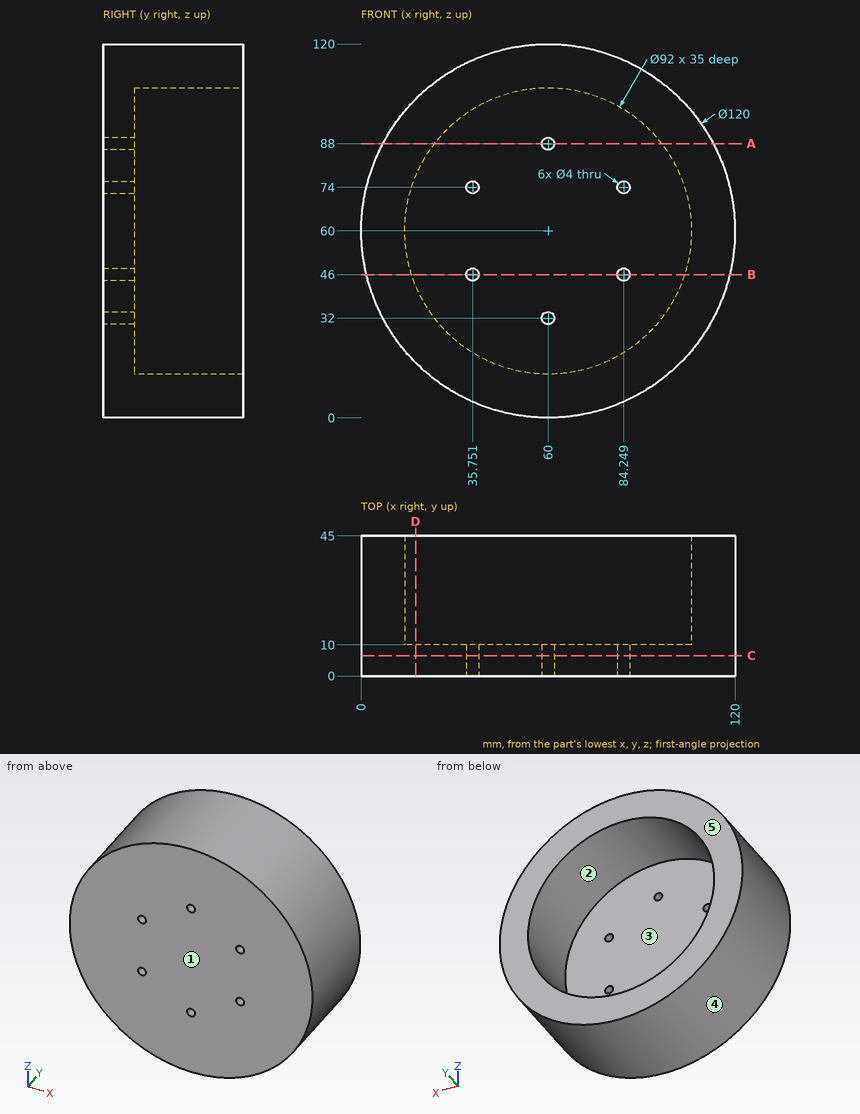
Print and shaded views of the part. All mm, measured from the part's lowest x, y and z. A direction names the side the tool comes from. Round coordinates to 2 decimals unless told otherwise and drop trailing zeros. Write each loop counter-clockwise with the first axis right and the second up, starting at its lowest first coordinate (ties: lowest second). Pieces come first, ordered by that corner, then holes. Notation, with made-up numbers: (87, 37.25) - (98, 37.25) arc R15 ccw to (98, 62.25) - close; hole circle Ø6 at (8.25, 46). An arc over 180 degrees is marked (long way). One line per item, written item: value.
(1) Cut at C-C, the plane y = 6.5. Give the cut face in (x, z), plus the area to 3 significant figures.
Values follow:
outline: circle Ø120 at (60, 60); hole circle Ø4 at (35.75, 46); hole circle Ø4 at (35.75, 74); hole circle Ø4 at (60, 32); hole circle Ø4 at (60, 88); hole circle Ø4 at (84.25, 46); hole circle Ø4 at (84.25, 74)
area: 11,200 mm²
(2) Drop flat-ended pins along their axis: P1, Ø3, axis at x = 60, z = 88, coming from the -Y side; P2, Ø4, axis at x = 36.5, z = 37, coming from the +Y side; P3, Ø1, axis at x = 80.5, y = 30, coming from the +Z side; P4, Ø1.5, axis at y = 32, z = 57.5, coming from the -X side. Give the stop position or say it passes through.
Values follow:
P1: passes through
P2: stops at y = 10
P3: stops at z = 116.57
P4: stops at x = 0.03
(3) Cut at D-D, the plane x = 17.5. Give the cut face in (y, z).
Values follow:
outline: (0, 17.65) - (45, 17.65) - (45, 42.4) - (10, 42.4) - (10, 77.6) - (45, 77.6) - (45, 102.35) - (0, 102.35) - close
(4) Cut at A-A, the plane z = 88. Give the cut face in (x, y), plus the area to 3 significant figures.
Values follow:
outline: (6.93, 0) - (58, 0) - (58, 10) - (23.5, 10) - (23.5, 45) - (6.93, 45) - close; (62, 0) - (113.07, 0) - (113.07, 45) - (96.5, 45) - (96.5, 10) - (62, 10) - close
area: 2,180 mm²
(5) Wall check: probe 1 along X at (y, z) = (5.5, 74); probe 2 along X at (y, z) = (28, 60); probe 3 along Y at (x, z) = (74.5, 37.5). Give the ranges that are in metal, low to high.
Values follow:
probe 1: x = 1.66 to 33.75, 37.75 to 82.25, 86.25 to 118.34
probe 2: x = 0 to 14, 106 to 120
probe 3: y = 0 to 10
(6) Two-plate mould, pull along Z, no slides. Class the marked faces 3, 4 and 5: pulls with the +Z half, pulls with the -Z half, needs draft (parallel to the pull), parting line crosses it, or undercut.
Values follow:
face 3: undercut
face 4: parting line crosses it
face 5: needs draft
(7) Cut at B-B, the plane z = 46. Give the cut face in (x, y).
Values follow:
outline: (1.66, 0) - (33.75, 0) - (33.75, 10) - (16.18, 10) - (16.18, 45) - (1.66, 45) - close; (37.75, 0) - (82.25, 0) - (82.25, 10) - (37.75, 10) - close; (86.25, 0) - (118.34, 0) - (118.34, 45) - (103.82, 45) - (103.82, 10) - (86.25, 10) - close
(8) 3-axis set-ups, long thin cutter, end or side, ignore diameter. For the marked faces 1 and 2: which of +Z, -Z, +X, -X, +Y, -Y reach the whole face in a straight line?
Values follow:
face 1: +Z, -Z, +X, -X, -Y
face 2: +Y
